Work out the finished part from the listing and answer in its coordinate system (mm). A direction names the side the tool comes from. Coordinates: 2 decimals unless noted, no trailing zeros. Order: outer loops, then holes, each group sorted by start corner. A loop starts at its lowest first (then second) coordinate and runs counter-clockwise, first axis right, second up.
1. Determine the mould class of faces 4 (the flat face through (-27, 0, 42)), 5 (the flat face through (51.5, 10, 23)) for opening direction Z: +Z half, -Z half, draft (parallel to the pull), parting line (faces both ways), or undercut.
2. The part is cut by section C-C, the plane y = 7.25. Give the vertices of the cut face in (x, z) (3 decimals), then the cut area to 3 significant figures.
3. Find the intervals of material crossed by probe 1 along Z at (x, y) = (42.5, 10.5); probe 2 along X at (y, z) = (10.25, -25); probe 3 along Z at (x, y) = (-42.5, 7), in increasing order.
4. The part is cut by section B-B, the plane x = 30. Give the vertices of the cut face in (y, z) (3 decimals), then the cut area to 3 significant figures.
5. The part is cut by section D-D, the plane z = -25. Give the vertices of the cut face in (x, y).
6. Flat-ended cylindrical pins translate along their axes: pin 1 Ø1.5 at (x, z) = (41, 23) entering from -Y; pin 2 Ø1.5 at (x, z) = (9, 9) entering from +Y; pin 3 Ø4 at (x, z) = (42.5, -25) entering from +Y. Find the tip coordinate at first contact, or state that the pin passes through.
7. The part is cut by section A-A, the plane z = 36. Give the vertices of the cut face in (x, y).
8. A tool of negligible diameter and unlimited length cuts with its end or side. For faces 1 (the cylindrical face through (44.94, 9.2, -24.46)), 2 (the flat face through (-51, 15, 3)), 3 (the flat face through (25, 2, 19.5)), from which of +Z, -Z, +X, -X, +Y, -Y can it reach the whole face along a straight path? Write none if from no direction.
```python
from build123d import *

# Parameters (mm, degrees)
SKETCH1_W               = 107
SKETCH1_H               = 87
BOSS_EXTRUDE1_DEPTH     = 13.92
SKETCH2_W               = 103
SKETCH2_H               = 83
CUT_EXTRUDE1_DEPTH      = 7.92
SKETCH3_R               = 2.5
BOSS_EXTRUDE2_DEPTH     = 6.5
CUT_EXTRUDE2_DEPTH      = 70.406241794
CUT_EXTRUDE2_DEPTH_BACK = 4
SKETCH4_R               = 1.2
SKETCH5_W               = 28
SKETCH5_H               = 4
CUT_EXTRUDE3_DEPTH      = 70.406241794
SKETCH6_W               = 2.5
SKETCH6_H               = 24
CUT_EXTRUDE4_DEPTH      = 70.406241794
SKETCH7_R               = 1.6
CUT_EXTRUDE6_DEPTH      = 70.406241794
SKETCH8_W               = 8
SKETCH8_H               = 7.92
CUT_EXTRUDE9_DEPTH      = 4
SKETCH9_W               = 1.5
SKETCH9_H               = 11.25
BOSS_EXTRUDE4_DEPTH     = 4.8
SKETCH10_W              = 1.5
SKETCH10_H              = 6
BOSS_EXTRUDE5_DEPTH     = 8.2
BOSS_EXTRUDE6_DEPTH     = 6
SKETCH12_W              = 103
SKETCH12_H              = 83
CUT_EXTRUDE10_DEPTH     = 4
SKETCH13_W              = 34.87
SKETCH13_H              = 4
CUT_EXTRUDE11_DEPTH     = 118.056610236
SKETCH14_W              = 28
SKETCH14_H              = 2.5
BOSS_EXTRUDE9_DEPTH     = 4
BOSS_EXTRUDE10_DEPTH    = 25
BOSS_EXTRUDE11_DEPTH    = 25
SKETCH16_W              = 15
SKETCH16_H              = 4
CUT_EXTRUDE12_DEPTH     = 104.885754558
BOSS_EXTRUDE12_DEPTH    = 4


with BuildPart() as part:
    # Sketch1 → Boss-Extrude1 (new body)
    with BuildSketch(Plane(origin=(0, 0, 0), x_dir=(1, 0, 0), z_dir=(0, 1, 0))):
        Rectangle(SKETCH1_W, SKETCH1_H)
    extrude(amount=BOSS_EXTRUDE1_DEPTH)

    # Sketch2 → Cut-Extrude1 (cut)
    with BuildSketch(Plane(origin=(0, 13.92, 0), x_dir=(1, 0, 0), z_dir=(0, 1, 0))):
        Rectangle(SKETCH2_W, SKETCH2_H)
    extrude(amount=-CUT_EXTRUDE1_DEPTH, mode=Mode.SUBTRACT)

    # Sketch3 → Boss-Extrude2 (add)
    with BuildSketch(Plane(origin=(0, 6, 0), x_dir=(1, 0, 0), z_dir=(0, 1, 0))):
        with Locations(Location((-42.5, -25, 0), (0, 0, 90))):
            Circle(SKETCH3_R)
        with Locations(Location((42.5, 25, 0), (0, 0, 90))):
            Circle(SKETCH3_R)
    extrude(amount=BOSS_EXTRUDE2_DEPTH)

    # Sketch4 → Cut-Extrude2 (cut, two sides: drawn at the far end of the back side and taken through both)
    with BuildSketch(Plane(origin=(0, 6, 0), x_dir=(1, 0, 0), z_dir=(0, 1, 0)).offset(-CUT_EXTRUDE2_DEPTH_BACK)):
        with Locations(Location((-42.5, -25, 0), (0, 0, 270))):
            Circle(SKETCH4_R)
        with Locations(Location((42.5, 25, 0), (0, 0, 270))):
            Circle(SKETCH4_R)
    extrude(amount=CUT_EXTRUDE2_DEPTH + CUT_EXTRUDE2_DEPTH_BACK, mode=Mode.SUBTRACT)

    # Sketch5 → Cut-Extrude3 (cut, through all)
    with BuildSketch(Plane(origin=(0, 6, 0), x_dir=(1, 0, 0), z_dir=(0, 1, 0))):
        with Locations((-34.36, 15)):
            Rectangle(SKETCH5_W, SKETCH5_H)
        with Locations((34.36, 15)):
            Rectangle(SKETCH5_W, SKETCH5_H)
    extrude(amount=-CUT_EXTRUDE3_DEPTH, mode=Mode.SUBTRACT)

    # Sketch6 → Cut-Extrude4 (cut, through all)
    with BuildSketch(Plane(origin=(0, 6, 0), x_dir=(1, 0, 0), z_dir=(0, 1, 0))):
        with Locations((6.25, -27.5)):
            Rectangle(SKETCH6_W, SKETCH6_H)
        with Locations((-6.25, -27.5)):
            Rectangle(SKETCH6_W, SKETCH6_H)
    extrude(amount=-CUT_EXTRUDE4_DEPTH, mode=Mode.SUBTRACT)

    # Sketch7 → Cut-Extrude6 (cut, through all)
    with BuildSketch(Plane(origin=(0, 6, 0), x_dir=(1, 0, 0), z_dir=(0, 1, 0))):
        with Locations(Location((-1, -23.8, 0), (0, 0, 270))):
            Circle(SKETCH7_R)
    extrude(amount=-CUT_EXTRUDE6_DEPTH, mode=Mode.SUBTRACT)

    # Sketch8 → Cut-Extrude9 (cut)
    with BuildSketch(Plane.ZY.offset(53.5)):
        with Locations((0, 9.96)):
            Rectangle(SKETCH8_W, SKETCH8_H)
    cut_extrude9 = extrude(amount=-CUT_EXTRUDE9_DEPTH, mode=Mode.SUBTRACT)

    # Sketch9 → Boss-Extrude4 (add)
    with BuildSketch(Plane(origin=(0, 6, 0), x_dir=(1, 0, 0), z_dir=(0, 1, 0))):
        with Locations((-50.75, 0)):
            Rectangle(SKETCH9_W, SKETCH9_H)
    boss_extrude4 = extrude(amount=BOSS_EXTRUDE4_DEPTH)

    # Sketch10 → Boss-Extrude5 (add)
    with BuildSketch(Plane(origin=(0, 10.8, 0), x_dir=(1, 0, 0), z_dir=(0, 1, 0))):
        with Locations((-50.75, 0)):
            Rectangle(SKETCH10_W, SKETCH10_H)
    boss_extrude5 = extrude(amount=BOSS_EXTRUDE5_DEPTH)

    # Sketch11 → Boss-Extrude6 (add)
    with BuildSketch(Plane.XY.offset(3)):
        Polygon((-51.5, 19), (-52.4, 17.5), (-52.4, 17), (-51.5, 17), align=None)
    boss_extrude6 = extrude(amount=-BOSS_EXTRUDE6_DEPTH)

    # Mirror2: Cut-Extrude9, Boss-Extrude4, Boss-Extrude5, Boss-Extrude6 across plane
    add(cut_extrude9.mirror(Plane(origin=(0, 0, 0), x_dir=(0, 0, 1), z_dir=(1, 0, 0))), mode=Mode.SUBTRACT)
    add(boss_extrude4.mirror(Plane(origin=(0, 0, 0), x_dir=(0, 0, 1), z_dir=(1, 0, 0))))
    add(boss_extrude5.mirror(Plane(origin=(0, 0, 0), x_dir=(0, 0, 1), z_dir=(1, 0, 0))))
    add(boss_extrude6.mirror(Plane(origin=(0, 0, 0), x_dir=(0, 0, 1), z_dir=(1, 0, 0))))

    # Sketch12 → Cut-Extrude10 (cut)
    with BuildSketch(Plane.XZ):
        Rectangle(SKETCH12_W, SKETCH12_H)
    extrude(amount=-CUT_EXTRUDE10_DEPTH, mode=Mode.SUBTRACT)

    # Sketch13 → Cut-Extrude11 (cut, through all)
    with BuildSketch(Plane.ZY.offset(53.5)):
        with Locations((0, 2)):
            Rectangle(SKETCH13_W, SKETCH13_H)
    cut_extrude11 = extrude(amount=-CUT_EXTRUDE11_DEPTH, mode=Mode.SUBTRACT)

    # Sketch14 → Boss-Extrude9 (add)
    with BuildSketch(Plane(origin=(0, 4, 0), x_dir=(-1, 0, 0), z_dir=(0, -1, 0))):
        with Locations((37.5, 18.685)):
            Rectangle(SKETCH14_W, SKETCH14_H)
    boss_extrude9 = extrude(amount=BOSS_EXTRUDE9_DEPTH)

    # Sketch15 → Boss-Extrude10 (add)
    with BuildSketch(Plane(origin=(-23.5, 0, 0), x_dir=(0, 0, -1), z_dir=(1, 0, 0))):
        Polygon((17.435, 0), (14.935, 0), (14.935, 1), (16.435, 2.5), (17.435, 2.5), align=None)
    boss_extrude10 = extrude(amount=-BOSS_EXTRUDE10_DEPTH)

    # Mirror8: Cut-Extrude11, Boss-Extrude9, Boss-Extrude10 across plane
    add(cut_extrude11.mirror(Plane(origin=(0, 0, 0), x_dir=(0, 0, 1), z_dir=(1, 0, 0))), mode=Mode.SUBTRACT)
    add(boss_extrude9.mirror(Plane(origin=(0, 0, 0), x_dir=(0, 0, 1), z_dir=(1, 0, 0))))
    add(boss_extrude10.mirror(Plane(origin=(0, 0, 0), x_dir=(0, 0, 1), z_dir=(1, 0, 0))))

    # Sketch15_2 → Boss-Extrude11 (add)
    with BuildSketch(Plane(origin=(-23.5, 0, 0), x_dir=(0, 0, -1), z_dir=(1, 0, 0))):
        Polygon((17.435, 0), (14.935, 0), (14.935, 1), (16.435, 2.5), (17.435, 2.5), align=None)
    extrude(amount=-BOSS_EXTRUDE11_DEPTH)

    # Sketch16 → Cut-Extrude12 (cut, through all)
    with BuildSketch(Plane.XY.offset(43.5)):
        with Locations((0, 2)):
            Rectangle(SKETCH16_W, SKETCH16_H)
    cut_extrude12 = extrude(amount=-CUT_EXTRUDE12_DEPTH, mode=Mode.SUBTRACT)

    # Sketch18 → Boss-Extrude12 (add)
    with BuildSketch(Plane(origin=(0, 4, 0), x_dir=(-1, 0, 0), z_dir=(0, -1, 0))):
        Polygon((7.5, -41.5), (7.5, -17.37), (39.5, -17.37), (43.5, -19.017333388), (42.75, -20.838458378), (39.5, -19.5), (10.5, -19.5), (10.5, -41.5), align=None)
    boss_extrude12 = extrude(amount=BOSS_EXTRUDE12_DEPTH)

    # Mirror9: Cut-Extrude12, Boss-Extrude12 across plane
    add(cut_extrude12.mirror(Plane(origin=(0, 0, 0), x_dir=(0, 0, 1), z_dir=(1, 0, 0))), mode=Mode.SUBTRACT)
    add(boss_extrude12.mirror(Plane(origin=(0, 0, 0), x_dir=(0, 0, 1), z_dir=(1, 0, 0))))


solid = part.part
```
Geometry says:
1. face 4: draft
1. face 5: undercut
2. outline: (-53.5, -43.5) - (53.5, -43.5) - (53.5, -4) - (51.5, -4) - (51.5, 4) - (53.5, 4) - (53.5, 43.5) - (-53.5, 43.5) - (-53.5, 4) - (-51.5, 4) - (-51.5, -4) - (-53.5, -4) - close; circle Ø5 at (-42.5, 25); circle Ø5 at (42.5, -25); hole (-51.5, -41.5) - (51.5, -41.5) - (51.5, -5.625) - (50, -5.625) - (50, 5.625) - (51.5, 5.625) - (51.5, 41.5) - (-51.5, 41.5) - (-51.5, 5.625) - (-50, 5.625) - (-50, -5.625) - (-51.5, -5.625) - close; hole circle Ø2.4 at (-42.5, 25); hole circle Ø2.4 at (42.5, -25)
2. area: 792 mm2
3. probe 1: z = -43.5 to -41.5, -27.5 to -26.2, -23.8 to -22.5, 41.5 to 43.5
3. probe 2: x = -53.5 to -51.5, 40 to 41.3, 43.7 to 45, 51.5 to 53.5
3. probe 3: z = -43.5 to -41.5, 22.5 to 23.8, 26.2 to 27.5, 41.5 to 43.5
4. outline: (0, -43.5) - (13.92, -43.5) - (13.92, -41.5) - (6, -41.5) - (6, -17) - (4, -17) - (4, -17.435) - (2.5, -17.435) - (2.5, -16.435) - (1, -14.935) - (0, -14.935) - (0, -19.935) - (4, -19.935) - (4, -41.5) - (0, -41.5) - close; (0, 17.37) - (4, 17.37) - (4, -13) - (6, -13) - (6, 41.5) - (13.92, 41.5) - (13.92, 43.5) - (0, 43.5) - (0, 41.5) - (4, 41.5) - (4, 19.5) - (0, 19.5) - close
4. area: 237 mm2
5. outline: (-53.5, 0) - (-51.5, 0) - (-51.5, 4) - (41.3, 4) - (41.3, 12.5) - (40, 12.5) - (40, 6) - (-51.5, 6) - (-51.5, 13.92) - (-53.5, 13.92) - close; (43.7, 4) - (51.5, 4) - (51.5, 0) - (53.5, 0) - (53.5, 13.92) - (51.5, 13.92) - (51.5, 6) - (45, 6) - (45, 12.5) - (43.7, 12.5) - close
6. pin 1: stops at y = 4
6. pin 2: stops at y = 6
6. pin 3: stops at y = 12.5
7. outline: (-53.5, 0) - (-51.5, 0) - (-51.5, 4) - (-10.5, 4) - (-10.5, 0) - (-7.5, 0) - (-7.5, 6) - (-51.5, 6) - (-51.5, 13.92) - (-53.5, 13.92) - close; (-5, 4) - (5, 4) - (5, 6) - (-5, 6) - close; (7.5, 0) - (10.5, 0) - (10.5, 4) - (51.5, 4) - (51.5, 0) - (53.5, 0) - (53.5, 13.92) - (51.5, 13.92) - (51.5, 6) - (7.5, 6) - close
8. face 1: +Y
8. face 2: +X, -X, +Y
8. face 3: -Y
